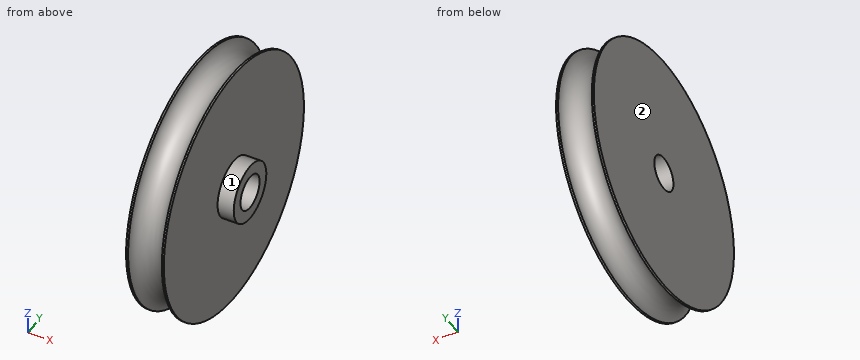
from build123d import *


with BuildPart() as f1:
    # F0 (on Front) → F1 (revolve)
    with BuildSketch(Plane.XZ):
        with BuildLine():
            Line((0, 23.8125), (0, 3.2512))
            Line((0, 3.2512), (10.16, 3.2512))
            Line((10.16, 3.2512), (10.16, 5.5372))
            Line((10.16, 5.5372), (7.112, 5.5372))
            Line((7.112, 5.5372), (7.112, 23.8125))
            Line((7.112, 23.8125), (6.731, 23.8125))
            ThreePointArc((6.731, 23.8125), (3.556, 20.6375), (0.381, 23.8125))
            Line((0.381, 23.8125), (0, 23.8125))
        make_face()
    revolve(axis=Axis((6.071118, 0, 0), (1, 0, 0)))


solid = f1.part
Model file for the job. Use its own axes, mm. Face numbers are marked on the shaded views. A direction names the side the tool comes from. Round coordinates to 2 decimals unless told otherwise and drop trailing zeros. Order: outer loops, then holes, each group sorted by start corner. A loop starts at its lowest first (then second) coordinate and runs counter-clockwise, first axis right, second up.
(1) Drill centre lines: line 1 (Z direction, x = 8.25, y = 0); line 2 (Z direction, x = 7, y = 0). Where is each one in solid material? Low to high.
(2) Pin check, flat tips, straight feed: pin 1 (6 mm diameter, centred on x = 8.5, y = -7, fed in from -Z); pin 2 (5 mm diameter, centred on x = 2, y = -3.5, fed in from +Z); pin 3 (8 mm diameter, centred on y = 17, z = -5.5, fed in from +X). Stop position of each tip, or through.
(3) Band-saw the part on C-C (x = 8.75). List the corners of the cut face in (y, z), then the cut area to 3 significant figures.
(4) Band-saw the part on D-D (x = 2.5). List the corners of the cut face in (y, z), then the cut area to 3 significant figures.
(5) 3-axis set-ups, long thin cutter, end or side, ignore diameter. For the marked faces 1 and 2: which of +Z, -Z, +X, -X, +Y, -Y reach the whole face in a straight line?
Verdict:
1. line 1: z = -5.54 to -3.25, 3.25 to 5.54
1. line 2: z = -23.81 to -3.25, 3.25 to 23.81
2. pin 1: stops at z = -23.41
2. pin 2: stops at z = 23.76
2. pin 3: stops at x = 7.11
3. outline: circle Ø11.07 at (0, 0); hole circle Ø6.5 at (0, 0)
3. area: 63.1 mm2
4. outline: circle Ø41.64 at (0, 0); hole circle Ø6.5 at (0, 0)
4. area: 1,330 mm2
5. face 1: +X
5. face 2: +Z, -Z, -X, +Y, -Y
